Autodesk Inventor part; units mm, degrees
ref_plane "YZ Plane" through (0, 0, 0) normal (1, 0, 0) x (0, 1, 0)
ref_plane "XZ Plane" through (0, 0, 0) normal (0, 1, 0) x (-1, 0, 0)
ref_plane "XY Plane" through (0, 0, 0) normal (0, 0, 1) x (1, 0, 0)
ref_plane "Płaszczyzna konstrukcyjna1" through (0, 0, 0) normal (0, 0, 1) x (1, 0, 0)
sketch "Szkic1" plane through (0, 0, 0) normal (0, 0, 1) x (1, 0, 0)
  circle A0 centre (0, 20) radius 2.5
  circle A1 centre (0, 35) radius 2.5
  circle A2 centre (0, 27.5) radius 40
  point P0 (0, 0)
  dimension "d0" = 7.5
  dimension "d1" = 7.5
  dimension "d2" = 80
extrude "Wyciągnięcie proste1" add sketch "Szkic1" along normal blind 3
chamfer "Faza1" distance 0.4 angle 45 2 edges at (-40, 27.5, 3) (-40, 27.5, 0)
chamfer "Faza3" distance 2 angle 45 2 edges at (-2.5, 20, 3) (-2.5, 35, 3)
sketch "Szkic2" plane through (0, 27.5, 0) normal (0, 0, -1) x (-1, 0, 0)
  circle A0 centre (0, 7.5) radius 2.5
  circle A1 centre (0, -7.5) radius 2.5
  circle A2 centre (0, -47.5) radius 2
  circle A3 centre (0, -62.5) radius 2
  line L0 (6.05, 12.2) -> (6.05, -67.2)
  line L1 (-6.05, 12.2) -> (6.05, 12.2)
  line L2 (-6.05, -67.2) -> (-6.05, 12.2)
  line L3 (6.05, -67.2) -> (-6.05, -67.2)
  circle A4 centre (0, 7.5) radius 2.5
  circle A5 centre (0, -7.5) radius 2.5
  circle A6 centre (0, -47.5) radius 2
  circle A7 centre (0, -62.5) radius 2
  line L4 (6.05, 12.2) -> (6.05, -67.2)
  line L5 (-6.05, 12.2) -> (6.05, 12.2)
  line L6 (-6.05, -67.2) -> (-6.05, 12.2)
  line L7 (6.05, -67.2) -> (-6.05, -67.2)
  line L8 (10, -41.5) -> (-10, -41.5)
  line L9 (-10, -41.5) -> (-10, -15.5)
  line L10 (-8, -13.5) -> (8, -13.5)
  line L11 (10, -15.5) -> (10, -41.5)
  line L12 (10, -41.5) -> (-10, -13.5) construction
  line L13 (-10, -41.5) -> (10, -13.5) construction
  arc A8 (-8, -13.5) -> (-10, -15.5) centre (-8, -15.5) ccw
  arc A9 (10, -15.5) -> (8, -13.5) centre (8, -15.5) ccw
  point P0 (0, -27.5)
  point P1 (0, -27.5)
  dimension "d14" = 20
  dimension "d15" = 28
  dimension "d16" = 20
  dimension "d17" = 2
extrude "Wyciągnięcie proste2" cut sketch "Szkic2" against normal blind 2 contours L10 A9 L11 L8 L0 | L0 L8 L2 L10 | L2 L8 L9 A8 L10
properties part number "szklo" material "Akrylowy, przezroczysty"
Could you check a few things on this model? Use its own coordinates, in mm. A direction names the side the tool comes from. Give positions to 0.01 mm unless a question says otherwise; leave off trailing zeros. Loops run counter-clockwise (first coordinate to the right, second up) from the corner with the lowest first, then second, coordinate; pieces in that order, holes last. Notation, with made-up numbers: (-33.75, -20) -> (-5.75, -20) arc R18 ccw to (-5.75, 2) -> close; hole circle Ø1 at (-10.75, -30). An arc over 180 degrees is marked (long way). Answer as CSV lines item,"result". Start each with the question number.
(1) We'd pull the mould along Y, two halves only. Please class faces 3 (the cylindrical face through (1.34, 17.89, 0.49)), 4 (the conical face through (1.61, 67.18, 0.11)), 5 (the flat face through (0, 14, 1)), 6 (the flat face through (-1, 29, 0)): released by +Y, released by -Y, zero draft, split by the parting line, or undercut.
(2) Which directions (+Z, -Z, +X, -X, +Y, -Y) give clear straight access to the entire face, cutting with the end or side of a thin tool? Please do faces 1 (the cylindrical face through (-8.67, 66.55, 1.48)), 2 (the flat face through (0, 1, 2)).
(3) I need wall thicknesses on probe 1 along Y at (x, z) = (0, 0.7); probe 2 along Y at (x, z) = (0, 0.3); probe 3 along X at (y, z) = (-4, 1.6). Which ranges of each line are inside material? Lowest first, please.
(4) I'm going to push flat-ended pins straight in: pin 1 Ø0.6 at (y, z) = (1.5, 1.5) entering from +X; pin 2 Ø2 at (x, y) = (24.5, 31.5) entering from -Z; pin 3 Ø6 at (x, y) = (0, 35) entering from +Z; pin 4 Ø1 at (x, y) = (-32, 0.5) entering from +Z. Where does each tip first touch, or does it pass through?
(5) If we section it at A-A on x = 0: Write out the boundary of the cut face in (y, z).
Computed:
1,face 3,"undercut"
1,face 4,"split by the parting line"
1,face 5,"released by -Y"
1,face 6,"zero draft"
2,face 1,"+Z, -Z"
2,face 2,"-Z, -Y"
3,probe 1,"y = 14 to 17.5, 22.5 to 32.5, 37.5 to 67.5"
3,probe 2,"y = 14 to 17.5, 22.5 to 32.5, 37.5 to 67.4"
3,probe 3,"x = -24.65 to -10, 10 to 24.65"
4,pin 1,"stops at x = 30.65"
4,pin 2,"stops at z = 0"
4,pin 3,"stops at z = 1.5"
4,pin 4,"passes through"
5,outline,"(-12.5, 2) -> (14, 2) -> (14, 0) -> (17.5, 0) -> (17.5, 1) -> (15.5, 3) -> (-12.1, 3) -> (-12.5, 2.6) -> close; (22.5, 0) -> (32.5, 0) -> (32.5, 1) -> (30.5, 3) -> (24.5, 3) -> (22.5, 1) -> close; (37.5, 0) -> (67.1, 0) -> (67.5, 0.4) -> (67.5, 2.6) -> (67.1, 3) -> (39.5, 3) -> (37.5, 1) -> close"
